Geometry: final body of the model. Coordinates: model frame, mm. A direction names the side the tool comes from. Coordinates: 2 decimals unless noted, no trailing zeros. Loops run counter-clockwise (first coordinate to the right, second up) from the corner with the lowest first, then second, coordinate; pieces in that order, holes last. Notation, with made-up numbers: (70.5, 33.5) - (113.5, 33.5) arc R22 ccw to (113.5, 67.5) - close; hole circle Ø4 at (41, -34). An arc over 180 degrees is marked (long way). Put each result on its own line as item: value. Start each with the question number.
1) Section D-D on z = 8. Count the separate pieces of the cut face and the enclosed holes in it, and give its area (3 significant figures).
2) Draft query along Y for faces 4 (the flat face through (7, 0, 5)), 5 (the flat face through (7, 4, 10)), 6 (the flat face through (15, 7.2, 7)), 7 (the flat face through (11, 7.2, 7)). Return one class per face: +Y half, -Y half, draft (parallel to the pull), parting line (faces both ways), or undercut.
3) Section C-C on x = 11. Output: boundary loops of the cut face in (y, z), and give its area (3 significant figures).
4) Reachability of faces 1 (the cylindrical face through (0.46, 27.1, 5.07)), 2 (the flat face through (9.5, 19.6, 6.5)), 3 (the flat face through (4, 20, 7)) from +Z, -Z, +X, -X, +Y, -Y: full face, straight path, thin tool, end or side. Return the list, or none.
5) Section A-A on z = 1. Output: boundary loops of the cut face in (x, y), and give its area (3 significant figures).
6) Material intervals for line 1 along Y through (x, z) = (7, 8.5); line 2 along Y through (x, z) = (13, 5.5); line 3 along Y through (x, z) = (12.5, 1.5), sorted ascending. Write a range as from..to.
7) Contact query for flat-ended pins moving along their axis: pin 1 Ø0.9 at (y, z) = (8, 5) entering from +X; pin 2 Ø1.3 at (x, z) = (1, 5.5) entering from +Y. Output: stop coordinate, or through.
```python
from build123d import *

# Parameters (mm, degrees)
BOX_W        = 19
BOX_H        = 1.1
BOX_DEPTH    = 7
SKETCH015_W  = 1.2
SKETCH015_H  = 7
PAD_DEPTH    = 0.8
BOX002_W     = 19
BOX002_H     = 1.1
BOX002_DEPTH = 7
SKETCH016_W  = 1.2
SKETCH016_H  = 7
PAD001_DEPTH = 0.8
BOX001_W     = 15.8
BOX001_H     = 28
BOX001_DEPTH = 10
FILLET_R     = 3


with BuildPart() as pad:
    # Box → Box (new body)
    with BuildSketch(Plane(origin=(-0.5, 20, 3.1), x_dir=(1, 0, 0), z_dir=(0, 0, 1))):
        with Locations((9.5, 0.55)):
            Rectangle(BOX_W, BOX_H)
    extrude(amount=BOX_DEPTH)

    # Sketch015 → Pad (new body)
    with BuildSketch(Plane(origin=(-0.5, 20, 3.1), x_dir=(1, 0, 0), z_dir=(0, -1, 0))):
        with Locations((1.4, 3.5)):
            Rectangle(SKETCH015_W, SKETCH015_H)
        with Locations((3.4, 3.5)):
            Rectangle(SKETCH015_W, SKETCH015_H)
        with Locations((5.4, 3.5)):
            Rectangle(SKETCH015_W, SKETCH015_H)
        with Locations((7.4, 3.5)):
            Rectangle(SKETCH015_W, SKETCH015_H)
        with Locations((9.4, 3.5)):
            Rectangle(SKETCH015_W, SKETCH015_H)
        with Locations((11.4, 3.5)):
            Rectangle(SKETCH015_W, SKETCH015_H)
        with Locations((13.4, 3.5)):
            Rectangle(SKETCH015_W, SKETCH015_H)
        with Locations((15.4, 3.5)):
            Rectangle(SKETCH015_W, SKETCH015_H)
    extrude(amount=PAD_DEPTH)


with BuildPart() as pad001:
    # Box002 → Box002 (new body)
    with BuildSketch(Plane(origin=(-0.5, 8, 3.1), x_dir=(1, 0, 0), z_dir=(0, 0, 1))):
        with Locations((9.5, 0.55)):
            Rectangle(BOX002_W, BOX002_H)
    extrude(amount=BOX002_DEPTH)

    # Sketch016 → Pad001 (new body)
    with BuildSketch(Plane(origin=(-0.5, 8, 3.1), x_dir=(1, 0, 0), z_dir=(0, -1, 0))):
        with Locations((1.4, 3.5)):
            Rectangle(SKETCH016_W, SKETCH016_H)
        with Locations((3.4, 3.5)):
            Rectangle(SKETCH016_W, SKETCH016_H)
        with Locations((5.4, 3.5)):
            Rectangle(SKETCH016_W, SKETCH016_H)
        with Locations((7.4, 3.5)):
            Rectangle(SKETCH016_W, SKETCH016_H)
        with Locations((9.4, 3.5)):
            Rectangle(SKETCH016_W, SKETCH016_H)
        with Locations((11.4, 3.5)):
            Rectangle(SKETCH016_W, SKETCH016_H)
        with Locations((13.4, 3.5)):
            Rectangle(SKETCH016_W, SKETCH016_H)
        with Locations((15.4, 3.5)):
            Rectangle(SKETCH016_W, SKETCH016_H)
    extrude(amount=PAD001_DEPTH)


with BuildPart() as fillet_body:
    # Box001 → Box001 (new body)
    with BuildSketch(Plane(origin=(-0.4, 0, 0), x_dir=(1, 0, 0), z_dir=(0, 0, 1))):
        with Locations((7.9, 14)):
            Rectangle(BOX001_W, BOX001_H)
    extrude(amount=BOX001_DEPTH)

    # Cut: cut Pad001
    add(pad001.part, mode=Mode.SUBTRACT)

    # Cut001: cut Pad
    add(pad.part, mode=Mode.SUBTRACT)

    # Fillet
    fillet_edges = [fillet_body.edges().sort_by_distance(p)[0] for p in [
        (-0.4, 28, 5),
        (-0.4, 0, 5),
        (15.4, 28, 5),
        (15.4, 0, 5),
    ]]
    fillet(fillet_edges, radius=FILLET_R)


solid = fillet_body.part
```
Answer block:
1. separate pieces: 3
1. enclosed holes: 0
1. area: 385 mm²
2. face 4: -Y half
2. face 5: draft
2. face 6: undercut
2. face 7: undercut
3. outline: (0, 0) - (28, 0) - (28, 10) - (21.1, 10) - (21.1, 3.1) - (19.2, 3.1) - (19.2, 10) - (9.1, 10) - (9.1, 3.1) - (7.2, 3.1) - (7.2, 10) - (0, 10) - close
3. area: 254 mm²
4. face 1: +Z, -Z, -X, +Y
4. face 2: +Z
4. face 3: +Z, +X, -X
5. outline: (-0.4, 3) arc R3 ccw to (2.6, 0) - (12.4, 0) arc R3 ccw to (15.4, 3) - (15.4, 25) arc R3 ccw to (12.4, 28) - (2.6, 28) arc R3 ccw to (-0.4, 25) - close
5. area: 435 mm²
6. line 1: y = 0..7.2, 9.1..19.2, 21.1..28
6. line 2: y = 0.06..7.2, 9.1..19.2, 21.1..27.94
6. line 3: y = 0..28
7. pin 1: stops at x = 14.3
7. pin 2: stops at y = 27.85
